Build history of the part. All positions in model axes, mm. A direction names the side the tool comes from. Round coordinates to 2 decimals unless told otherwise and drop trailing zeros. Loops run counter-clockwise (first coordinate to the right, second up) from the corner with the lowest first, then second, coordinate; pieces in that order, holes last.
Autodesk Inventor part; units mm, degrees
ref_plane "YZ Plane" through (0, 0, 0) normal (1, 0, 0) x (0, 1, 0)
ref_plane "XZ Plane" through (0, 0, 0) normal (0, 1, 0) x (-1, 0, 0)
ref_plane "XY Plane" through (0, 0, 0) normal (0, 0, 1) x (1, 0, 0)
sketch "Sketch1" plane through (0, 0, 0) normal (0, 1, 0) x (-1, 0, 0)
  arc A0 (9, -28.6182) -> (-9, -28.6182) centre (0, 0) ccw
  arc A1 (-3, 39.8873) -> (-3, -39.8873) centre (0, 0) ccw construction
  line L0 (0, 0) -> (-200, 0) construction
  arc A2 (-175, 0) -> (-200, 25) centre (-200, 0) ccw construction
  line L1 (-200, 25) -> (-200, -25) construction
  line L2 (-3, -39.8873) -> (-201.875, -24.9296)
  line L3 (-3, 39.8873) -> (-201.875, 24.9296)
  arc A3 (-3, -39.8873) -> (-3, 39.8873) centre (0, 0) ccw
  arc A4 (-200, -25) -> (-175, 0) centre (-200, 0) ccw construction
  arc A5 (-200, 25) -> (-200, -25) centre (-200, 0) ccw
  line L4 (0, 0) -> (0, -30) construction
  line L5 (9, -23) -> (-9, -23) construction
  line L6 (9, -23) -> (9, -28.6182) construction
  line L7 (-9, -23) -> (-9, -28.6182) construction
  line L8 (9, -28.6182) -> (9, -34)
  line L9 (-9, -28.6182) -> (-9, -34)
  line L10 (9, -34) -> (-9, -34)
  arc A6 (0, -30) -> (9, -28.6182) centre (0, 0) ccw construction
  arc A7 (-9, -28.6182) -> (0, -30) centre (0, 0) ccw construction
  dimension "d0" = 60
  dimension "d1" = 80
  dimension "d2" = 200
  dimension "d3" = 50
  dimension "d5" = 18
  dimension "d6" = 7
  dimension "d7" = 4
extrude "Extrusion1" add sketch "Sketch1" along normal blind 25
sketch "Sketch2" plane through (0, 25, 0) normal (0, 1, 0) x (1, 0, 0)
  arc A0 (201.875, -24.9296) -> (201.875, 24.9296) centre (200, 0) ccw
  circle A1 centre (200, 0) radius 9.525
  point P0 (0, 0)
  dimension "d10" = 19.05
extrude "Extrusion4" cut sketch "Sketch2" against normal through all
sketch "Sketch4" plane through (-9, 0, -34) normal (0, 0, 1) x (1, 0, 0)
  line L0 (0, 0) -> (18, 0)
  line L1 (18, 0) -> (18, 25)
  line L2 (0, 25) -> (18, 25)
  line L3 (0, 0) -> (0, 25)
  line L4 (9, 25) -> (9, 0) construction
  line L5 (0, 0) -> (0, 25) construction
  line L6 (0, 12.5) -> (18, 12.5) construction
  circle A0 centre (9, 12.5) radius 7.9375
  dimension "d24" = 15.875
extrude "Extrusion5" cut sketch "Sketch4" against normal blind 10 contours A0
properties part number "placa manivela" material "Steel, Carbon"
(1) Slice it at C-C on z = 12.5. List the corners of the cut face in (x, y), plus the area to 3 significant figures.
Responses:
outline: (-38, 0) - (-27.27, 0) - (-27.27, 25) - (-38, 25) - close; (27.27, 0) - (221.65, 0) - (221.65, 25) - (27.27, 25) - close
area: 5,130 mm2
(2) Pull direction Y, two halves, no side cores. Call faces 1 (the face through (224.995, 12.325, -0.523)), 2 (the face through (94, 25, 1)), 3 (the face through (7.332, 9.46, -36.958)), 4 (the face through (94, 0, 1)): +Y half, -Y half, draft (parallel to the pull), parting line (faces both ways), or undercut.
Responses:
face 1: draft
face 2: +Y half
face 3: undercut
face 4: -Y half
(3) Slice it at B-B on z = 0. List the corners of the cut face in (x, y) (3 decimals), plus the area to 3 significant figures.
Responses:
outline: (-40, 0) - (-30, 0) - (-30, 25) - (-40, 25) - close; (30, 0) - (190.475, 0) - (190.475, 25) - (30, 25) - close; (209.525, 0) - (225, 0) - (225, 25) - (209.525, 25) - close
area: 4,650 mm2
(4) Pin check, flat tips, straight feed: P1, Ø2, axis at y = 16.5, z = -6.5, coming from the -X side; P2, Ø4, axis at y = 20, z = -12, coming from the +X side; P3, Ø1.6, axis at y = 7.5, z = -30.5, coming from the -X side. Stop position of each tip, or through.
Responses:
P1: stops at x = -39.62
P2: stops at x = 222.91
P3: stops at x = -26.79
(5) Probe line 1 (Y direction, x = 0, z = -38.35); line 2 (Z direction, x = -20, y = 16); line 3 (Z direction, x = -17, y = 15.5). List the from-to ranges inside material, lowest first.
Responses:
line 1: y = 0 to 4.56, 20.44 to 25
line 2: z = -34.64 to -22.36, 22.36 to 34.64
line 3: z = -36.21 to -24.72, 24.72 to 36.21
(6) Slice it at A-A on x = 0. List the corners of the cut face in (y, z).
Responses:
outline: (0, -40) - (4.56, -40) - (4.56, -34) - (0, -34) - close; (0, 30) - (25, 30) - (25, 40) - (0, 40) - close; (20.44, -40) - (25, -40) - (25, -34) - (20.44, -34) - close
(7) Which spindle directions (+Z, -Z, +X, -X, +Y, -Y) get a long thin tool onto all of the face, cutting with end or side? Do faces 5 (the face through (101.045, 12.325, 32.513)), 6 (the face through (9, 12, -31)). Say none if no direction does.
Responses:
face 5: +Z, +X, +Y, -Y
face 6: +Y, -Y
(8) Slice it at D-D on x = 198. List the corners of the cut face in (y, z).
Responses:
outline: (0, -25.22) - (25, -25.22) - (25, -9.31) - (0, -9.31) - close; (0, 9.31) - (25, 9.31) - (25, 25.22) - (0, 25.22) - close
